```python
from build123d import *

# Parameters (mm, degrees)
BOSS_EXTRUDE1_DEPTH     = 2
SKETCH2_R               = 1.6
SKETCH2_R_2             = 7.5
CUT_EXTRUDE1_DEPTH      = 3
SKETCH3_R               = 1.5
SKETCH3_W               = 20
SKETCH3_H               = 1
CUT_EXTRUDE2_DEPTH      = 1
CUT_EXTRUDE2_DEPTH_BACK = 3


with BuildPart() as part:
    # Sketch1 → Boss-Extrude1 (new body)
    with BuildSketch(Plane.XY):
        Polygon((76, 28.5), (-76, 28.5), (-76, 5), (-74, 5), (-74, -5), (-76, -5), (-76, -28.5), (76, -28.5), (76, -5), (74, -5), (74, 5), (76, 5), align=None)
    extrude(amount=BOSS_EXTRUDE1_DEPTH)

    # Sketch2 → Cut-Extrude1 (cut, through all)
    with BuildSketch(Plane.XY.offset(2)):
        with Locations((-72.5, 24.05)):
            Circle(SKETCH2_R)
        with Locations((72.5, 24.05)):
            Circle(SKETCH2_R)
        with Locations((66, -24.05)):
            Circle(SKETCH2_R)
        with Locations((-66, -24.05)):
            Circle(SKETCH2_R)
        with Locations((-56, 0)):
            Circle(SKETCH2_R_2)
    extrude(amount=-CUT_EXTRUDE1_DEPTH, mode=Mode.SUBTRACT)

    # Sketch3 → Cut-Extrude2 (cut, two sides)
    with BuildSketch(Plane.XY.offset(2)) as cut_extrude2_sk:
        with Locations((32, -14.95)):
            Circle(SKETCH3_R)
        with Locations((-56, 15.05)):
            Circle(SKETCH3_R)
        with Locations((-56, -14.95)):
            Circle(SKETCH3_R)
        with Locations((32, 15.05)):
            Circle(SKETCH3_R)
        with Locations((-44, 28)):
            Rectangle(SKETCH3_W, SKETCH3_H)
    extrude(amount=CUT_EXTRUDE2_DEPTH, mode=Mode.SUBTRACT)
    extrude(cut_extrude2_sk.sketch, amount=-CUT_EXTRUDE2_DEPTH_BACK, mode=Mode.SUBTRACT)


solid = part.part
```
The listing builds one solid part. Answer for the finished solid, in the listing's coordinates (mm). Round coordinates to 2 decimals unless told otherwise and drop trailing zeros. Order: outer loops, then holes, each group sorted by start corner. A loop starts at its lowest first (then second) coordinate and runs counter-clockwise, first axis right, second up. Notation, with made-up numbers: (-39, -12.75) - (18, -12.75) arc R24 cw to (18, 1.25) - close; hole circle Ø5 at (-20, 39). An arc over 180 degrees is marked (long way). Put each result on its own line as item: value. Start each with the question number.
(1) Find section C-C (z = 1). State how many separate pieces and enclosed holes the cut face has, plus the area to 3 significant figures.
(2) Find section A-A (x = -56). Give the vertices of the cut face in (y, z), plus the area to 3 significant figures.
(3) Straight lines are drawn through the part: probe 1 along Y at (x, z) = (32, 1.65); probe 2 along Y at (x, z) = (-56, 1.5); probe 3 along Y at (x, z) = (-57, 0.75). For each, find the intervals that lie inside material, in ascending order. Write a range as from..to.
(4) Given P1, Ø2.5, axis at x = -72.5, y = 24.05, coming from the +Z side; P2, Ø3.5, axis at x = 32, y = -14.95, coming from the -Z side; P3, Ø0.6, axis at x = -40, z = 0.5, coming from the +Y side, each flat-ended and moving along its own axis, determine where each tip first touches the part or whether it passes through.
(5) Find section B-B (x = 66). Give the vertices of the cut face in (y, z).
(6) Determine the mould class of faces 1 (the flat face through (-1, 0, 0)), 2 (the cylindrical face through (30.81, -15.86, 1.01)) for opening direction Y: released by +Y, released by -Y, zero draft, split by the parting line, or undercut.
(7) Find section D-D (x = 32). Give the vertices of the cut face in (y, z).
Reply:
1. separate pieces: 1
1. enclosed holes: 9
1. area: 8,370 mm^2
2. outline: (-28.5, 0) - (-16.45, 0) - (-16.45, 2) - (-28.5, 2) - close; (-13.45, 0) - (-7.5, 0) - (-7.5, 2) - (-13.45, 2) - close; (7.5, 0) - (13.55, 0) - (13.55, 2) - (7.5, 2) - close; (16.55, 0) - (28.5, 0) - (28.5, 2) - (16.55, 2) - close
2. area: 72.0 mm^2
3. probe 1: -28.5..-16.45, -13.45..13.55, 16.55..28.5
3. probe 2: -28.5..-16.45, -13.45..-7.5, 7.5..13.55, 16.55..28.5
3. probe 3: -28.5..-16.07, -13.83..-7.43, 7.43..13.93, 16.17..28.5
4. P1: through
4. P2: z = 0
4. P3: y = 27.5
5. outline: (-28.5, 0) - (-25.65, 0) - (-25.65, 2) - (-28.5, 2) - close; (-22.45, 0) - (28.5, 0) - (28.5, 2) - (-22.45, 2) - close
6. face 1: zero draft
6. face 2: undercut
7. outline: (-28.5, 0) - (-16.45, 0) - (-16.45, 2) - (-28.5, 2) - close; (-13.45, 0) - (13.55, 0) - (13.55, 2) - (-13.45, 2) - close; (16.55, 0) - (28.5, 0) - (28.5, 2) - (16.55, 2) - close
